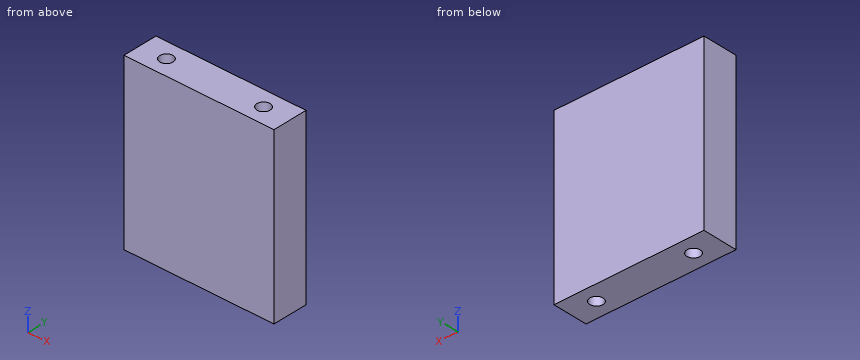
from build123d import *

# Parameters (mm, degrees)
SKETCH1_W           = 107.95
SKETCH1_H           = 25.4
BOSS_EXTRUDE1_DEPTH = 123.65
SKETCH2_R           = 4.7625
SKETCH2_R_2         = 4.765
CUT_EXTRUDE1_DEPTH  = 25.4


with BuildPart() as part:
    # Sketch1 → Boss-Extrude1 (new body)
    with BuildSketch(Plane.XY):
        with Locations((53.975, -12.7)):
            Rectangle(SKETCH1_W, SKETCH1_H)
    extrude(amount=BOSS_EXTRUDE1_DEPTH)

    # Sketch2 → Cut-Extrude1 (cut)
    with BuildSketch(Plane.XY.offset(123.65)):
        with Locations((19.05, -12.7)):
            Circle(SKETCH2_R)
        with Locations((88.9, -12.7)):
            Circle(SKETCH2_R_2)
    cut_extrude1 = extrude(amount=-CUT_EXTRUDE1_DEPTH, mode=Mode.SUBTRACT)

    # Mirror1: Cut-Extrude1 across plane
    add(cut_extrude1.mirror(Plane.XY.offset(61.825)), mode=Mode.SUBTRACT)


solid = part.part
Geometry check sheet. Reference: the model listing, model coordinates, mm. Round coordinates to 2 decimals unless told otherwise and drop trailing zeros. Order: outer loops, then holes, each group sorted by start corner. A loop starts at its lowest first (then second) coordinate and runs counter-clockwise, first axis right, second up. Notation, with made-up numbers: (-3.75, 42) -> (25.25, 42) arc R15 cw to (25.25, 50) -> close; hole circle Ø7 at (-1, -18). An arc over 180 degrees is marked (long way). Use one line per item in the form item = value.
1. Cross-section at A-A, the plane x = 88.9. Enter the section's corners in (y, z) (3 decimals).
Working result:
outline = (-25.4, 0) -> (-17.465, 0) -> (-17.465, 25.4) -> (-7.935, 25.4) -> (-7.935, 0) -> (0, 0) -> (0, 123.65) -> (-7.935, 123.65) -> (-7.935, 98.25) -> (-17.465, 98.25) -> (-17.465, 123.65) -> (-25.4, 123.65) -> close
2. Scan lines: line 1 along Y through (x, z) = (19.05, 12); line 2 along X through (y, z) = (-10, 9); line 3 along X through (y, z) = (-16.25, 98.5). Record each from-to range of solid material in increasing order. Write a range as from..to.
Working result:
line_1 = -25.4..-17.46, -7.94..0
line_2 = 0..15.13, 22.97..84.97, 92.83..107.95
line_3 = 0..15.88, 22.22..85.72, 92.08..107.95
3. Go/stop test with flat-tipped pins: pin 1 (7.5 mm diameter, centred on x = 19.05, y = -12.7, fed in from -Z); pin 2 (3 mm diameter, centred on x = 87, y = -12, fed in from +Z). Record where each tip stops, or that it passes through.
Working result:
pin_1 = 25.4
pin_2 = 98.25
4. Cross-section at C-C, the plane x = 19.05. Enter the section's corners in (y, z), plus the area to 3 significant figures.
Working result:
outline = (-25.4, 0) -> (-17.46, 0) -> (-17.46, 25.4) -> (-7.94, 25.4) -> (-7.94, 0) -> (0, 0) -> (0, 123.65) -> (-7.94, 123.65) -> (-7.94, 98.25) -> (-17.46, 98.25) -> (-17.46, 123.65) -> (-25.4, 123.65) -> close
area = 2,660 mm^2
